Here's how the part is built. I have some questions about the finished solid (model axes, mm). A direction names the side the tool comes from. Give positions to 0.01 mm unless a question says otherwise; leave off trailing zeros. Write each loop counter-clockwise with the first axis right and the second up, starting at its lowest first coordinate (ties: lowest second). Pieces come first, ordered by that corner, then holes. Notation, with made-up numbers: (26, 55.5) - (48, 55.5) arc R9 cw to (48, 68.5) - close; hole circle Ø4 at (-18, 11). An arc over 180 degrees is marked (long way). One line per item, written item: value. Start each with the question number.
1) Imagine slicing it at A-A on z = -23.5. Write out the boundary of the cut face in (x, y).
2) I'm going to push a flat-ended pin straight in: P1, Ø3, axis at x = 23.5, z = -23.5, coming from the -Y side. Where does the tip first touch, or does it pass through?
3) Imagine slicing it at B-B on x = -23.5. Write out the boundary of the cut face in (y, z), plus the area to 3 significant figures.
4) Imagine slicing it at C-C on y = 1.65. Write out the boundary of the cut face in (x, z).
5) On a 3-axis mill with a long thin cutter (end or side, diameter ignored), from which of +Z, -Z, +X, -X, +Y, -Y can I reach the whole of each face in a straight line? I mean faces 4 (the flat face through (8.65, 1, 24)), 5 (the cylindrical face through (-22.532, 0.986, 21.982)). Say none if no direction works.
6) Please list where these lines run through material, in increasing order: L1, parallel to X at y = 0.4, z = 23.5; L2, parallel to X at y = 1.4, z = -23.5; L3, parallel to Z at x = 23, y = 0.8. Write a range as [from, to].
7) We'd pull the mould along Z, two halves only. Please class faces 1 (the cylindrical face through (24.468, 0.986, 21.982)), 2 (the flat face through (20.65, 1, 24)), 3 (the flat face through (15, 1, 21.5)): +Z half, -Z half, draft (parallel to the pull), parting line (faces both ways), or undercut.
8) Imagine slicing it at D-D on z = 23.5. Write out the boundary of the cut face in (x, y).
from build123d import *

# Parameters (mm, degrees)
SKETCH_3_R      = 1.8
EXTRUDE_2_DEPTH = 2


with BuildPart() as part:
    # 草图3 → 凸台-拉伸2 (new body)
    with BuildSketch(Plane(origin=(0, 0, 0), x_dir=(1, 0, 0), z_dir=(0, 1, 0))):
        Polygon((27, 27), (-27, 27), (-27, -27), (8.65, -27), (8.65, -21.5), (20.65, -21.5), (20.65, -27), (27, -27), align=None)
        with Locations((-23.5, -23.5)):
            Circle(SKETCH_3_R, mode=Mode.SUBTRACT)
        with Locations((23.5, -23.5)):
            Circle(SKETCH_3_R, mode=Mode.SUBTRACT)
        with Locations((-23.5, 23.5)):
            Circle(SKETCH_3_R, mode=Mode.SUBTRACT)
        with Locations((23.5, 23.5)):
            Circle(SKETCH_3_R, mode=Mode.SUBTRACT)
    extrude(amount=EXTRUDE_2_DEPTH)


solid = part.part
Numbers:
1. outline: (-27, 0) - (-25.3, 0) - (-25.3, 2) - (-27, 2) - close; (-21.7, 0) - (21.7, 0) - (21.7, 2) - (-21.7, 2) - close; (25.3, 0) - (27, 0) - (27, 2) - (25.3, 2) - close
2. P1: through
3. outline: (0, -27) - (2, -27) - (2, -25.3) - (0, -25.3) - close; (0, -21.7) - (2, -21.7) - (2, 21.7) - (0, 21.7) - close; (0, 25.3) - (2, 25.3) - (2, 27) - (0, 27) - close
3. area: 93.6 mm^2
4. outline: (-27, -27) - (27, -27) - (27, 27) - (20.65, 27) - (20.65, 21.5) - (8.65, 21.5) - (8.65, 27) - (-27, 27) - close; hole circle Ø3.6 at (-23.5, -23.5); hole circle Ø3.6 at (-23.5, 23.5); hole circle Ø3.6 at (23.5, -23.5); hole circle Ø3.6 at (23.5, 23.5)
5. face 4: +Z, +Y, -Y
5. face 5: +Y, -Y
6. L1: [-27, -25.3], [-21.7, 8.65], [20.65, 21.7], [25.3, 27]
6. L2: [-27, -25.3], [-21.7, 21.7], [25.3, 27]
6. L3: [-27, -25.23], [-21.77, 21.77], [25.23, 27]
7. face 1: undercut
7. face 2: draft
7. face 3: +Z half
8. outline: (-27, 0) - (-25.3, 0) - (-25.3, 2) - (-27, 2) - close; (-21.7, 0) - (8.65, 0) - (8.65, 2) - (-21.7, 2) - close; (20.65, 0) - (21.7, 0) - (21.7, 2) - (20.65, 2) - close; (25.3, 0) - (27, 0) - (27, 2) - (25.3, 2) - close
